Could you check a few things on this model? Use its own coordinates, in mm. A direction names the side the tool comes from. Round coordinates to 2 decimals unless told otherwise and drop trailing zeros. Loops run counter-clockwise (first coordinate to the right, second up) from the corner with the lowest first, then second, coordinate; pieces in that order, holes last. Notation, with made-up numbers: (-13, -10) - (-3, -10) arc R25 cw to (-3, 28) - close; hole circle Ø9 at (-20, 71). An arc over 180 degrees is marked (long way). Put each result on its own line as item: value. Start each with the question number.
from build123d import *

# Parameters (mm, degrees)
F1_DEPTH    = 5
F2_SIZE     = 1
F3_T1_DEPTH = 5
F4_R        = 0.1


# Not quite as in the source:
# - a fillet or chamfer that OpenCascade refuses, or shapes differently, is made with other operations: its cross-section is extruded or revolved along the edge and cut away or added


with BuildPart() as f1:
    # F0 (on Front) → F1 (new body)
    with BuildSketch(Plane.XZ):
        with BuildLine():
            ThreePointArc((0.5760859311, -0.625), (-0.8390441156, -0.1360329819), (0.3491060011, 0.775))
            Line((0.3491060011, 0.775), (2.2185299187, 0.775))
            Line((2.2185299187, 0.775), (2.2185299187, 2.0197594836))
            Line((2.2185299187, 2.0197594836), (6.65, 2.0197594836))
            Line((6.65, 2.0197594836), (6.65, 4.8197594836))
            Line((6.65, 4.8197594836), (5, 4.8197594836))
            Line((5, 4.8197594836), (5, 3.5197594836))
            Line((5, 3.5197594836), (0, 3.5197594836))
            Line((0, 3.5197594836), (0, 7.5197594836))
            Line((0, 7.5197594836), (5, 7.5197594836))
            Line((5, 7.5197594836), (5, 6.2197594836))
            Line((5, 6.2197594836), (6.65, 6.2197594836))
            Line((6.65, 6.2197594836), (6.65, 9.0197594836))
            Line((6.65, 9.0197594836), (-2.35, 9.0197594836))
            Line((-2.35, 9.0197594836), (-2.35, 0.4335492267))
            Line((-2.35, 0.4335492267), (-1.6366346435, 0))
            Line((-1.6366346435, 0), (-2.3136941642, -0.4114842822))
            ThreePointArc((-2.3136941642, -0.4114842822), (-0.1293198619, -2.2532607786), (2.2185299187, -0.625))
            Line((2.2185299187, -0.625), (0.5760859311, -0.625))
        make_face()
    extrude(amount=F1_DEPTH)

    # F2
    f2_edges = [f1.edges().sort_by_distance(p)[0] for p in [
        (6.65, -2.5, 6.219759),
        (6.65, -2.5, 4.819759),
    ]]
    chamfer(f2_edges, length=F2_SIZE)

    # F3: fillet of radius 5 on 1 edges, made by hand

    # F3_s2 → F3_t1 (join)
    with BuildSketch(Plane.XZ):
        with BuildLine():
            ThreePointArc((5.5197673631, 2.0197594836), (3.7557099068, 1.6982315944), (2.2185299187, 0.775))
            Line((2.2185299187, 0.775), (2.2185299187, 2.0197594836))
            Line((2.2185299187, 2.0197594836), (5.5197673631, 2.0197594836))
        make_face()
    extrude(amount=F3_T1_DEPTH)

    # F4
    f4_edges = [f1.edges().sort_by_distance(p)[0] for p in [
        (-1.636635, -2.5, 0),
        (-2.313694, -2.5, -0.411484),
        (-2.35, -2.5, 0.433549),
        (2.21853, -2.5, -0.625),
        (2.21853, -2.5, 0.775),
    ]]
    fillet(f4_edges, radius=F4_R)


solid = f1.part
Item 1: Suppose I cut it at B-B, the plane z = 6.5. List the corners of the cut face in (x, y) for me, then the cut area to 3 significant figures.
Item 2: Thinking about a two-plate mould opening in Z: for faces 1 (the face through (6.65, -2, 3)), 2 (the face through (1, -2, -0.625)), 3 (the face through (-0.21, -2.46, -2.25)), which applies, released by +Z, released by -Z, zero draft, split by the parting line, or undercut?
Item 3: Suppose I cut it at C-C, the plane x = 4. List the corners of the cut face in (y, z) for me.
Item 4: Will these pins go through, and if not, where does the flat tip stop? P1, Ø1.5, axis at x = 1.5, y = -3.5, coming from the -Z side; P2, Ø3, axis at x = 3, y = -3, coming from the -Z side.
Item 5: On a 3-axis mill with a long thin cutter (end or side, diameter ignored), from which of +Z, -Z, +X, -X, +Y, -Y can I reach the whole of each face in a straight line? I mean faces 4 (the face through (6, -2, 2.02)), 5 (the face through (6.14, -2.47, 4.33)), 6 (the face through (5, -2, 7)). Say none if no direction works.
Item 6: I need wall thicknesses on line 1 (Z direction, x = 1, y = -2.25) (3 decimals); line 2 (Z direction, x = 0.75, y = -4.8) (3 decimals); line 3 (X direction, y = -3.4, z = 0). Which ranges of each line are inside material? Lowest first, please. Write a range as from..to.
Item 7: Suppose I cut it at D-D, the plane x = -1.5. List the corners of the cut face in (y, z) for me, then the cut area to 4 significant figures.
Numbers:
1. outline: (-2.35, -5) - (0, -5) - (0, 0) - (-2.35, 0) - close; (5, -5) - (5.93, -5) - (5.93, 0) - (5, 0) - close
1. area: 16.4 mm^2
2. face 1: zero draft
2. face 2: undercut
2. face 3: released by -Z
3. outline: (-5, 1.78) - (0, 1.78) - (0, 3.52) - (-5, 3.52) - close; (-5, 7.52) - (0, 7.52) - (0, 9.02) - (-5, 9.02) - close
4. P1: z = -2.13
4. P2: z = -1.7
5. face 4: -Z, +X, +Y, -Y
5. face 5: +X, +Y, -Y
5. face 6: +Y, -Y
6. line 1: -2.024..-0.625, 0.775..3.52, 7.52..9.02
6. line 2: -2.127..-0.625, 0.775..3.52, 7.52..9.02
6. line 3: -1.73..-0.85
7. outline: (-5, -1.73) - (0, -1.73) - (0, 9.02) - (-5, 9.02) - close
7. area: 53.75 mm^2
